Check sheet for the drawn part. Datum: minimum x, y, z corner. Units: mm. Give positions to 0.01 mm unless a question says otherwise; leave off trailing zeros. Loops run counter-clockwise (first coordinate to the right, second up) from the corner with the lowest first, then second, coordinate; pieces in that order, holes last. Notation, with made-up numbers: (89.5, 88.5) - (139.5, 88.5) arc R8 ccw to (139.5, 95.5) - close; hole circle Ø5 at (22, -17). An arc over 180 degrees is marked (long way). One line per item, written item: value. Start each with the question number.
1. Sectioned sample at D-D (z = 4.35). Record the cut outline in (x, y), plus the area to 3 significant figures.
2. Gauge pin test, flat ends, axial feed: pin 1 (1.8 mm diameter, centred on x = 24, z = 3, fed in from +Y); pin 2 (3.5 mm diameter, centred on x = 10, y = 110, fed in from -Z). Record the tip position at first contact, or that the pin passes through.
3. Sectioned sample at A-A (x = 90). Record the cut outline in (y, z), plus the area to 3 significant figures.
4. Sectioned sample at B-B (y = 10). Record the cut outline in (x, z).
5. Sectioned sample at C-C (y = 79.5). Record the cut outline in (x, z).
6. Scan lines: L1, parallel to X at y = 102, z = 1.5; L2, parallel to Y at x = 10, z = 3.9; L3, parallel to Y at x = 55, z = 3.75. Record each from-to range of solid material in increasing order. Write a range as [from, to].
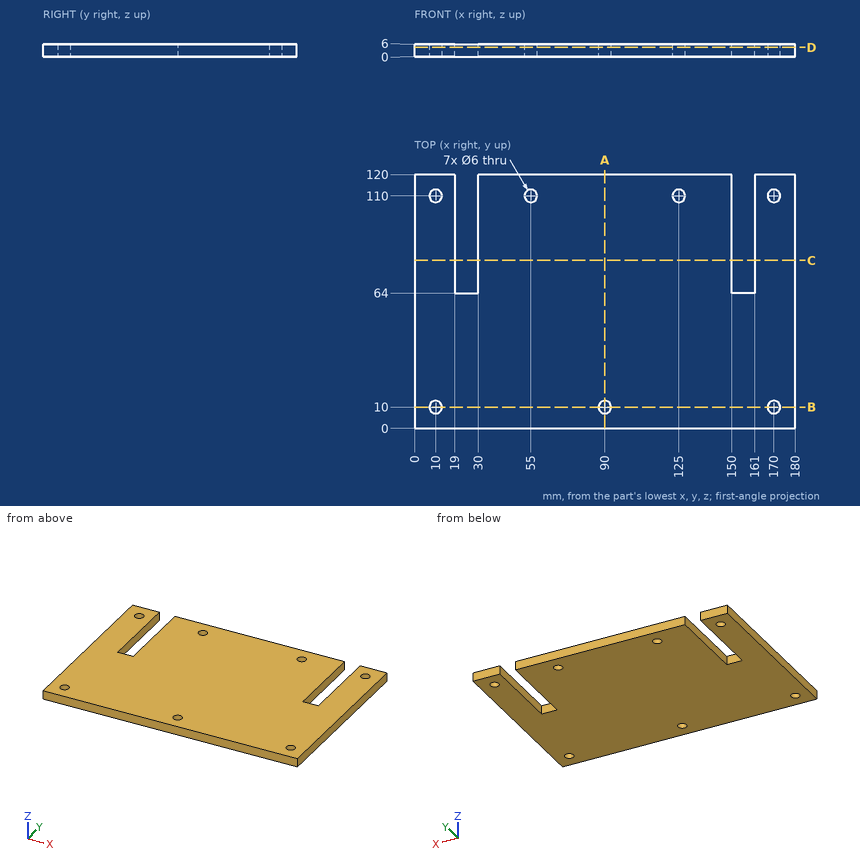
Results are:
1. outline: (0, 0) - (180, 0) - (180, 120) - (161, 120) - (161, 64) - (150, 64) - (150, 120) - (30, 120) - (30, 64) - (19, 64) - (19, 120) - (0, 120) - close; hole circle Ø6 at (10, 10); hole circle Ø6 at (10, 110); hole circle Ø6 at (55, 110); hole circle Ø6 at (90, 10); hole circle Ø6 at (125, 110); hole circle Ø6 at (170, 10); hole circle Ø6 at (170, 110)
1. area: 20,200 mm^2
2. pin 1: stops at y = 64
2. pin 2: passes through
3. outline: (0, 0) - (7, 0) - (7, 6) - (0, 6) - close; (13, 0) - (120, 0) - (120, 6) - (13, 6) - close
3. area: 684 mm^2
4. outline: (0, 0) - (7, 0) - (7, 6) - (0, 6) - close; (13, 0) - (87, 0) - (87, 6) - (13, 6) - close; (93, 0) - (167, 0) - (167, 6) - (93, 6) - close; (173, 0) - (180, 0) - (180, 6) - (173, 6) - close
5. outline: (0, 0) - (19, 0) - (19, 6) - (0, 6) - close; (30, 0) - (150, 0) - (150, 6) - (30, 6) - close; (161, 0) - (180, 0) - (180, 6) - (161, 6) - close
6. L1: x = [0, 19], [30, 150], [161, 180]
6. L2: y = [0, 7], [13, 107], [113, 120]
6. L3: y = [0, 107], [113, 120]
